```python
from build123d import *

# Parameters (mm, degrees)
F0_W     = 40.005
F0_H     = 40.005
F1_DEPTH = 3.175
F2_W     = 24.6475
F2_H     = 2.54
F3_DEPTH = 1.27


with BuildPart() as f1:
    # F0 (on Top) → F1 (new body)
    with BuildSketch(Plane.XY):
        Polygon((-44.65, -20.0025), (-44.65, -56.5), (44.65, -56.5), (44.65, 56.5), (-44.65, 56.5), (-44.65, 20.0025), (-44.65, 17.4625), (-44.65, -17.4625), align=None)
        Rectangle(F0_W, F0_H, mode=Mode.SUBTRACT)
    extrude(amount=F1_DEPTH)

    # F2 (on face) → F3 (cut)
    with BuildSketch(Plane(origin=(0, 0, 0), x_dir=(1, 0, 0), z_dir=(0, 0, -1))):
        with Locations((-32.32625, 18.7325)):
            Rectangle(F2_W, F2_H)
        with Locations((-32.32625, -18.7325)):
            Rectangle(F2_W, F2_H)
    extrude(amount=-F3_DEPTH, mode=Mode.SUBTRACT)


solid = f1.part
```
Model file for the job. Use its own axes, mm. A direction names the side the tool comes from. Give positions to 0.01 mm unless a question says otherwise; leave off trailing zeros. Loops run counter-clockwise (first coordinate to the right, second up) from the corner with the lowest first, then second, coordinate; pieces in that order, holes last. Notation, with made-up numbers: (71, 74) - (114, 74) arc R24 cw to (114, 107) - close; hole circle Ø7 at (22, 24.5). An arc over 180 degrees is marked (long way). One line per item, written item: value. Start each with the question number.
1. Slice it at C-C (z = 2.65). List the corners of the cut face in (x, y).
2. Pull direction X, two halves, no side cores. Call faces 1 (the flat face through (-20.002, 0, 2)), 2 (the flat face through (1, 56.5, 2)), 3 (the flat face through (44.65, -1, 2)): pulls with the +X half, pulls with the -X half, needs draft (parallel to the pull), parting line crosses it, or undercut.
3. Pin check, flat tips, straight feed: pin 1 (1.3 mm diameter, centred on x = -35, y = -18, fed in from -Z); pin 2 (1.3 mm diameter, centred on x = -33, y = 19, fed in from -Z). Stop position of each tip, or through.
4. Slice it at D-D (x = -36.5). List the corners of the cut face in (y, z) (1 decimal), plus the area to 3 significant figures.
5. Probe L1, parallel to Y at x = -26, z = 1; L2, parallel to Y at x = 9, z = 2.8; L3, parallel to X at y = -3, z = 2.05. List the from-to ranges inside material, lowest first. Write a range as from..to.
6. Which spindle directions (+Z, -Z, +X, -X, +Y, -Y) get a long thin tool onto all of the face, cutting with end or side? Do faces 4 (the flat face through (-6, -20.002, 2)), 5 (the flat face through (-32, 19, 1.27)), 6 (the flat face through (20.002, 0, 2)). Say none if no direction does.
7. Slice it at A-A (x = -18). List the corners of the cut face in (y, z) (1 decimal).
Solution:
1. outline: (-44.65, -56.5) - (44.65, -56.5) - (44.65, 56.5) - (-44.65, 56.5) - close; hole (-20, -20) - (20, -20) - (20, 20) - (-20, 20) - close
2. face 1: undercut
2. face 2: needs draft
2. face 3: pulls with the +X half
3. pin 1: stops at z = 0
3. pin 2: stops at z = 1.27
4. outline: (-56.5, 0) - (-20, 0) - (-20, 1.3) - (-17.5, 1.3) - (-17.5, 0) - (17.5, 0) - (17.5, 1.3) - (20, 1.3) - (20, 0) - (56.5, 0) - (56.5, 3.2) - (-56.5, 3.2) - close
4. area: 352 mm^2
5. L1: y = -56.5..-20, -17.46..17.46, 20..56.5
5. L2: y = -56.5..-20, 20..56.5
5. L3: x = -44.65..-20, 20..44.65
6. face 4: -Z
6. face 5: -Z, -X
6. face 6: +Z, -Z
7. outline: (-56.5, 0) - (-20, 0) - (-20, 3.2) - (-56.5, 3.2) - close; (20, 0) - (56.5, 0) - (56.5, 3.2) - (20, 3.2) - close
